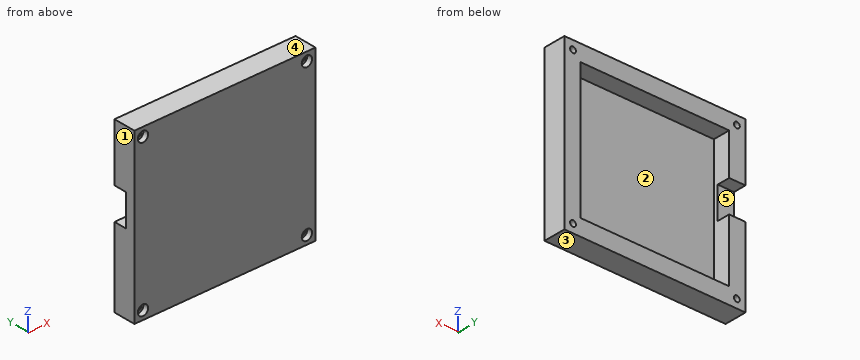
Autodesk Inventor part; units mm, degrees
ref_plane "YZ Plane" through (0, 0, 0) normal (1, 0, 0) x (0, 1, 0)
ref_plane "XZ Plane" through (0, 0, 0) normal (0, 1, 0) x (-1, 0, 0)
ref_plane "XY Plane" through (0, 0, 0) normal (0, 0, 1) x (1, 0, 0)
sketch "Sketch3" plane through (0, 0, 0) normal (0, 1, 0) x (-1, 0, 0)
  line L0 (0, 0) -> (86.5, 0)
  line L1 (86.5, 0) -> (86.5, -79.12)
  line L2 (86.5, -79.12) -> (0, -79.12)
  line L3 (0, -79.12) -> (0, 0)
  line L4 (-9.5, 9.5) -> (96, 9.5)
  line L5 (96, 9.5) -> (96, -88.62)
  line L6 (96, -88.62) -> (-9.5, -88.62)
  line L7 (-9.5, -88.62) -> (-9.5, 9.5)
  circle A0 centre (-4.5, 4.5) radius 1.7
  circle A1 centre (91, 4.5) radius 1.7
  circle A2 centre (-4.5, -83.62) radius 1.7
  circle A3 centre (91, -83.62) radius 1.7
  circle A4 centre (91, 4.5) radius 3
  circle A5 centre (-4.5, 4.5) radius 3
  circle A6 centre (-4.5, -83.62) radius 3
  circle A7 centre (91, -83.62) radius 3
  dimension "d0" = 86.5
  dimension "d1" = 79.12
  dimension "d2" = 105.5
  dimension "d3" = 98.12
  dimension "d4" = 9.5
  dimension "d5" = 9.5
  dimension "d6" = 3.4
  dimension "d7" = 3.4
  dimension "d8" = 3.4
  dimension "d9" = 3.4
  dimension "d10" = 5
  dimension "d11" = 5
  dimension "d12" = 5
  dimension "d13" = 5
  dimension "d14" = 5
  dimension "d15" = 5
  dimension "d16" = 5
  dimension "d17" = 5
  dimension "d18" = 6
  dimension "d19" = 6
  dimension "d20" = 6
  dimension "d21" = 6
extrude "Extrusion1" add sketch "Sketch3" along normal blind 13 contours A4 | A5 | A6 | A7
sketch "Sketch4" plane through (-91, 13, 4.5) normal (0, 1, 0) x (1, 0, 0)
  point P0 (91, 4.5)
extrude "Extrusion2" cut sketch "Sketch3" along normal blind 3.1 contours A4 | A5 | A6 | A7
extrude "Extrusion3" add sketch "Sketch3" along normal blind 13 contours L4 L5 L6 L7
extrude "Extrusion4" add sketch "Sketch3" along normal blind 3 contours L0 L1 L2 L3
sketch "Sketch6" plane through (0, 13, 0) normal (0, 1, 0) x (1, 0, 0)
  line L0 (-96, 88.62) -> (-96, -9.5)
  line L1 (-96, 24.122) -> (-86.5, 24.122)
  line L2 (-86.5, 24.122) -> (-86.5, 42.622)
  line L3 (-86.5, 42.622) -> (-96, 42.622)
  line L4 (-96, 42.622) -> (-96, 24.122)
  point P0 (0, 0)
  dimension "d31" = 9.5
  dimension "d32" = 18.5
extrude "Extrusion5" cut sketch "Sketch6" against normal blind 7.5
properties part number "Bottom_Plate"
The listing builds one solid part. Answer for the finished solid, in the listing's coordinates (mm). Face numbers are marked on the shaded views. A direction names the side the tool comes from. Round coordinates to 2 decimals unless told otherwise and drop trailing zeros. Loops run counter-clockwise (first coordinate to the right, second up) from the corner with the lowest first, then second, coordinate; pieces in that order, holes last. Notation, with made-up numbers: (17, 87) - (76, 87) arc R26 ccw to (76, 118) - close; hole circle Ø4 at (20.5, 69.25). An arc over 180 degrees is marked (long way). Use one line per item in the form item = value. Start each with the question number.
1. For a pull along X with two mould halves and no side action, classify the marked faces 1, 2 and 3 as pulls with the +X half, pulls with the -X half, needs draft (parallel to the pull), parting line crosses it, or undercut.
2. The part is cut by section A-A on x = -91. Determine the outline of the cut face in (y, z), then the cut area to 3 significant figures.
3. The part is cut by section D-D on z = -5.5. Determine the outline of the cut face in (x, y).
4. A tool of negligible diameter and unlimited length cuts with its end or side. For the marked faces 4 and 5, from which of +Z, -Z, +X, -X, +Y, -Y can it reach the whole face along a straight path? Write none if from no direction.
5. The part is cut by section B-B on z = 4.5. Determine the outline of the cut face in (x, y).
6. Consider line 1 (X direction, y = 11.25, z = -83.62); line 2 (Z direction, x = -91, y = 1.55); line 3 (Z direction, x = -91, y = 7.75). Determine where each line is inside the solid, lowest interval first. Write a range as [from, to].
7. Given pin 1 Ø4 at (x, z) = (-67, -14) entering from +Y; pin 2 Ø5 at (x, z) = (-91, 4.5) entering from +Y; pin 3 Ø4.5 at (x, z) = (4.5, -83.62) entering from -Y; pin 4 Ø2 at (x, z) = (4.5, 4.5) entering from -Y, each flat-ended and moving along its own axis, determine where each tip first touches the part or whether it passes through.
8. The part is cut by section C-C on y = 9. Determine the outline of the cut face in (x, z), then the cut area to 3 significant figures.
Geometry check:
q1.face_1 = pulls with the -X half
q1.face_2 = undercut
q1.face_3 = needs draft
q2.outline = (0, -88.62) - (13, -88.62) - (13, -85.32) - (3.1, -85.32) - (3.1, -86.62) - (0, -86.62) - close; (0, -80.62) - (3.1, -80.62) - (3.1, -81.92) - (13, -81.92) - (13, -42.62) - (5.5, -42.62) - (5.5, -24.12) - (13, -24.12) - (13, 2.8) - (3.1, 2.8) - (3.1, 1.5) - (0, 1.5) - close; (0, 7.5) - (3.1, 7.5) - (3.1, 6.2) - (13, 6.2) - (13, 9.5) - (0, 9.5) - close
q2.area = 1,030 mm^2
q3.outline = (-96, 0) - (9.5, 0) - (9.5, 13) - (0, 13) - (0, 3) - (-86.5, 3) - (-86.5, 13) - (-96, 13) - close
q4.face_4 = +Z, +X, -X, +Y, -Y
q4.face_5 = -X, +Y
q5.outline = (-96, 0) - (-94, 0) - (-94, 3.1) - (-92.7, 3.1) - (-92.7, 13) - (-96, 13) - close; (-89.3, 3.1) - (-88, 3.1) - (-88, 0) - (1.5, 0) - (1.5, 3.1) - (2.8, 3.1) - (2.8, 13) - (-89.3, 13) - close; (6.2, 3.1) - (7.5, 3.1) - (7.5, 0) - (9.5, 0) - (9.5, 13) - (6.2, 13) - close
q6.line_1 = [-96, -92.7], [-89.3, 2.8], [6.2, 9.5]
q6.line_2 = [-88.62, -86.62], [-80.62, 1.5], [7.5, 9.5]
q6.line_3 = [-88.62, -85.32], [-81.92, -42.62], [-24.12, 2.8], [6.2, 9.5]
q7.pin_1 = 3
q7.pin_2 = 13
q7.pin_3 = 3.1
q7.pin_4 = through
q8.outline = (-96, -88.62) - (9.5, -88.62) - (9.5, 9.5) - (-96, 9.5) - (-96, -24.12) - (-86.5, -24.12) - (-86.5, 0) - (0, 0) - (0, -79.12) - (-86.5, -79.12) - (-86.5, -42.62) - (-96, -42.62) - close; hole circle Ø3.4 at (-91, -83.62); hole circle Ø3.4 at (-91, 4.5); hole circle Ø3.4 at (4.5, -83.62); hole circle Ø3.4 at (4.5, 4.5)
q8.area = 3,300 mm^2
